```python
from build123d import *

# Parameters (mm, degrees)
F1_DEPTH = 100
F2_R     = 2
F3_R     = 1.9191209756
F4_DEPTH = 90
F5_R     = 1.25
F6_DEPTH = 20


# Not quite as in the source:
# - a feature names something its author has since deleted; it is built from what else it names


with BuildPart() as f1:
    # F0 (on Right) → F1 (new body)
    with BuildSketch(Plane.YZ):
        Polygon((2.3094010768, 4), (-2.3094010768, 4), (-4.6188021535, 0), (-2.3094010768, -4), (2.3094010768, -4), (4.6188021535, 0), align=None)
    extrude(amount=F1_DEPTH)

    # F2
    f2_edges = [f1.edges().sort_by_distance(p)[0] for p in [
        (50, -2.309401, 4),
        (50, -4.618802, 0),
        (50, -2.309401, -4),
        (50, 2.309401, 4),
        (50, 4.618802, 0),
        (50, 2.309401, -4),
    ]]
    fillet(f2_edges, radius=F2_R)

    # F3 (on face) → F4 (cut)
    with BuildSketch(Plane.YZ.offset(100)):
        Circle(F3_R)
    extrude(amount=-F4_DEPTH, mode=Mode.SUBTRACT)

    # F5 (on face) → F6 (cut)
    with BuildSketch(Plane.YZ.offset(10)):
        Circle(F5_R)
    extrude(amount=-F6_DEPTH, mode=Mode.SUBTRACT)


solid = f1.part
```
Check sheet for the modelled part. Datum: model origin and axes. Units: mm. Coordinates: 2 decimals unless noted, no trailing zeros. Write each loop counter-clockwise with the first axis right and the second up, starting at its lowest first coordinate (ties: lowest second). Pieces come first, ordered by that corner, then holes. Notation, with made-up numbers: (42.25, 41.25) -> (72.25, 41.25) arc R21 ccw to (72.25, 71.25) -> close; hole circle Ø3 at (86, 79.25). An arc over 180 degrees is marked (long way). Use a Markdown table: item, result.
1. Sectioned sample at B-B (z = 0). Enter the section's corners in (x, y), plus the area to 3 significant figures.
Reported:
| item | result |
|---|---|
| outline | (0, -4.31) -> (100, -4.31) -> (100, -1.92) -> (10, -1.92) -> (10, -1.25) -> (0, -1.25) -> close; (0, 1.25) -> (10, 1.25) -> (10, 1.92) -> (100, 1.92) -> (100, 4.31) -> (0, 4.31) -> close |
| area | 491 mm2 |
2. Release check for a two-part mould opening along Z. For faces 1 (the flat face through (49.3, 3.46, -2.01)), 2 (the cylindrical face through (50.7, 2.14, 3.74)), 3 (the cylindrical face through (55.63, 1.83, 0.58)), 4 (the cylindrical face through (5.07, -0.27, -1.22)) record: pulls with the +Z half, pulls with the -Z half, needs draft (parallel to the pull), parting line crosses it, or undercut.
Reported:
| item | result |
|---|---|
| face 1 | pulls with the -Z half |
| face 2 | pulls with the +Z half |
| face 3 | undercut |
| face 4 | undercut |
3. Go/stop test with flat-tipped pins: pin 1 Ø1.5 at (x, z) = (61.5, 1) entering from +Y; pin 2 Ø3 at (x, z) = (78, -2) entering from -Y. Record where each tip stops, or that it passes through.
Reported:
| item | result |
|---|---|
| pin 1 | stops at y = 4.29 |
| pin 2 | stops at y = -4.25 |
4. Sectioned sample at A-A (x = 43). Enter the section's corners in (y, z), plus the area to 3 significant figures.
Reported:
| item | result |
|---|---|
| outline | (-4.04, -1) -> (-2.89, -3) arc R2 ccw to (-1.15, -4) -> (1.15, -4) arc R2 ccw to (2.89, -3) -> (4.04, -1) arc R2 ccw to (4.04, 1) -> (2.89, 3) arc R2 ccw to (1.15, 4) -> (-1.15, 4) arc R2 ccw to (-2.89, 3) -> (-4.04, 1) arc R2 ccw to start; hole circle Ø3.84 at (0, 0) |
| area | 42.6 mm2 |
5. Sectioned sample at C-C (y = 0). Enter the section's corners in (x, z), plus the area to 3 significant figures.
Reported:
| item | result |
|---|---|
| outline | (0, -4) -> (100, -4) -> (100, -1.92) -> (10, -1.92) -> (10, -1.25) -> (0, -1.25) -> close; (0, 1.25) -> (10, 1.25) -> (10, 1.92) -> (100, 1.92) -> (100, 4) -> (0, 4) -> close |
| area | 430 mm2 |
6. Scan lines: line 1 along Z through (x, y) = (7, 0); line 2 along Z through (x, y) = (40.5, 0); line 3 along Y through (x, z) = (31.5, 0.5). Record each from-to range of solid material in increasing order.
Reported:
| item | result |
|---|---|
| line 1 | z = -4 to -1.25, 1.25 to 4 |
| line 2 | z = -4 to -1.92, 1.92 to 4 |
| line 3 | y = -4.25 to -1.85, 1.85 to 4.25 |
